Geometry: final body of the model. Coordinates: model frame, mm. A direction names the side the tool comes from. Give positions to 0.01 mm unless a question says otherwise; leave off trailing zeros. Order: outer loops, then holes, each group sorted by start corner. A loop starts at its lowest first (then second) coordinate and runs counter-clockwise, first axis right, second up. Notation, with made-up numbers: M 14.5,5.25 L 21.5,5.25 A27 cw 21.5,42.25 Z; hole C 48.5,37 d4. An arc over 180 degrees is marked long. One line per item, written item: value. Start each with the question number.
```python
from build123d import *

# Parameters (mm, degrees)
F3_R      = 9.525
F4_DEPTH  = 6.35
F6_R      = 12.7
F8_R      = 8.89
F9_DEPTH  = 101.6
F10_R     = 5.715
F11_DEPTH = 25.4
F13_R     = 9.525
F15_R     = 5.715
F16_DEPTH = 25.4


# Not quite as in the source:
# - a pattern or mirror of a feature is missing from the dataset's text; its kind, count and spacing are read off the source's solid


with BuildPart() as f1:
    # F0 (on Front) → F1 (revolve)
    with BuildSketch(Plane.XZ):
        with BuildLine():
            Line((-27.94, 0), (-41.275, 0))
            Line((-41.275, 0), (-41.275, -6.35))
            Line((-41.275, -6.35), (-31.75, -6.35))
            Line((-31.75, -6.35), (-31.75, -57.15))
            ThreePointArc((-31.75, -57.15), (-26.1703841816, -70.6203841816), (-12.7, -76.2))
            Line((-12.7, -76.2), (0, -76.2))
            Line((0, -76.2), (0, -72.39))
            Line((0, -72.39), (-12.7, -72.39))
            ThreePointArc((-12.7, -72.39), (-23.4763073453, -67.9263073453), (-27.94, -57.15))
            Line((-27.94, -57.15), (-27.94, 0))
        make_face()
    revolve(axis=Axis((0, 0, -38.1), (0, 0, 1)))



with BuildPart() as f2:
    # F0 (on Front) → F2 (revolve)
    with BuildSketch(Plane.XZ):
        with BuildLine():
            Line((-27.94, 0), (-41.275, 0))
            Line((-41.275, 0), (-41.275, -6.35))
            Line((-41.275, -6.35), (-31.75, -6.35))
            Line((-31.75, -6.35), (-31.75, -57.15))
            ThreePointArc((-31.75, -57.15), (-26.1703841816, -70.6203841816), (-12.7, -76.2))
            Line((-12.7, -76.2), (0, -76.2))
            Line((0, -76.2), (0, -72.39))
            Line((0, -72.39), (-12.7, -72.39))
            ThreePointArc((-12.7, -72.39), (-23.4763073453, -67.9263073453), (-27.94, -57.15))
            Line((-27.94, -57.15), (-27.94, 0))
        make_face()
    revolve(axis=Axis((0, 0, -38.1), (0, 0, 1)))


with BuildPart() as f1_1:
    add(f1.part)

    add(f2.part)  # F4 merges F2
    # F3 (on face) → F4 (join)
    with BuildSketch(Plane(origin=(0, 0, -76.2), x_dir=(1, 0, 0), z_dir=(0, 0, -1))):
        Circle(F3_R)
    extrude(amount=F4_DEPTH)

    # F6 (on offset) → F7 (join, up to the next surface of F1)
    with BuildSketch(Plane.XZ.offset(44.45)):
        with Locations((0, -31.75)):
            Circle(F6_R)
    f7 = extrude(until=Until.NEXT, dir=(0, 1, 0))

    # F7_copies: F7 across plane
    add(f7.mirror(Plane.ZX))

    # F8 (on face) → F9 (cut)
    with BuildSketch(Plane.XZ.offset(44.45)):
        with Locations((0, -31.75)):
            Circle(F8_R)
    extrude(amount=-F9_DEPTH, mode=Mode.SUBTRACT)

    # F10 (on face) → F11 (cut)
    with BuildSketch(Plane(origin=(0, 0, -82.55), x_dir=(1, 0, 0), z_dir=(0, 0, -1))):
        Circle(F10_R)
    extrude(amount=-F11_DEPTH, mode=Mode.SUBTRACT)

    # F13 (on offset) → F14 (join, up to the next surface of F1)
    with BuildSketch(Plane.YZ.offset(39.37)):
        with Locations((0, -31.75)):
            Circle(F13_R)
    extrude(until=Until.NEXT, dir=(-1, 0, 0))

    # F15 (on face) → F16 (cut)
    with BuildSketch(Plane.YZ.offset(39.37)):
        with Locations((0, -31.75)):
            Circle(F15_R)
    extrude(amount=-F16_DEPTH, mode=Mode.SUBTRACT)


solid = f1_1.part
```
Q1. Set-up query: faces 5 (the face through (34.89, -2.06, -41.05)), 6 (the face through (-26.65, -8.39, -28.17)), 7 (the face through (-21.2, 24.3, -6.35)), 8 (the face through (-5, -9, -76.2)). Return all of +Z, -Z, +X, -X, +Y, -Y with unobstructed straight access to the full face (end or side cutting, diameter ignored); none if empty.
Q2. Section query D-D on y = 0. Give the number of separate pieces and of enclosed holes in the cut face, and give its area (3 significant figures).
Q3. Section query C-C on x = 33.5. Return loops of the section in (y, z) (3 decimals), and give its area (3 significant figures).
Q4. Contact query for flat-ended pins moving along their axis: pin 1 (1.5 mm diameter, centred on x = -17.5, z = -36.5, fed in from +Y); pin 2 (1 mm diameter, centred on y = 4, z = -30.5, fed in from +X); pin 3 (6 mm diameter, centred on x = -21.5, y = 0, fed in from -Z). Output: stop coordinate, or through.
Q5. Section query B-B on z = -31.75. Return loops of the section in (x, y) (3 decimals).
Q6. Mould query, pull axis X, two halves, no side actions, for faces 1 (the face through (8.948, 40.293, -3.219)), 2 (the face through (0, 6, -82.55)), 3 (the face through (39.37, 6, -32)), 4 (the face through (-8.88, 35.34, -31.36)). Classes: +X half, -X half, draft (parallel to the pull), parting line (faces both ways), or undercut.
Q7. Section query A-A on y = 37. Return loops of the section in (x, z), and give its area (3 significant figures).
Q8. Ray query, line 1 along Z through (x, y) = (0, 40.75); line 2 along Y through (x, z) = (0, -16.5); line 3 along Z through (x, y) = (35, 0) (3 decimals). Return the intervals inside material, ascending. Write a range as [from, to].
Results below:
1. face 5: +X
1. face 6: +Z
1. face 7: none
1. face 8: -Z
2. separate pieces: 3
2. enclosed holes: 0
2. area: 878 mm2
3. outline: M -24.112,-6.35 L 24.112,-6.35 L 24.112,0 L -24.112,0 Z; C 0,-31.75 d19.05; hole C 0,-31.75 d11.43
3. area: 489 mm2
4. pin 1: y = 26.97
4. pin 2: x = -27.58
4. pin 3: z = -75.3
5. outline: M -12.7,-44.45 L -8.89,-44.45 L -8.89,-26.488 A27.94 cw -8.89,26.488 L -8.89,44.45 L -12.7,44.45 L -12.7,29.099 A31.75 ccw -12.7,-29.099 Z; M 8.89,-44.45 L 12.7,-44.45 L 12.7,-29.099 A31.75 ccw 30.288,-9.525 L 39.37,-9.525 L 39.37,-5.715 L 27.349,-5.715 A27.94 cw 8.89,-26.488 Z; M 8.89,26.488 A27.94 cw 27.349,5.715 L 39.37,5.715 L 39.37,9.525 L 30.288,9.525 A31.75 ccw 12.7,29.099 L 12.7,44.45 L 8.89,44.45 Z
6. face 1: parting line
6. face 2: draft
6. face 3: +X half
6. face 4: undercut
7. outline: M -18.29,-6.35 L 18.29,-6.35 L 18.29,0 L -18.29,0 Z; C 0,-31.75 d25.4; hole C 0,-31.75 d17.78
7. area: 491 mm2
8. line 1: [-44.45, -40.64], [-22.86, -19.05], [-6.35, 0]
8. line 2: [-31.75, -27.94], [27.94, 31.75]
8. line 3: [-41.275, -37.465], [-26.035, -22.225], [-6.35, 0]
